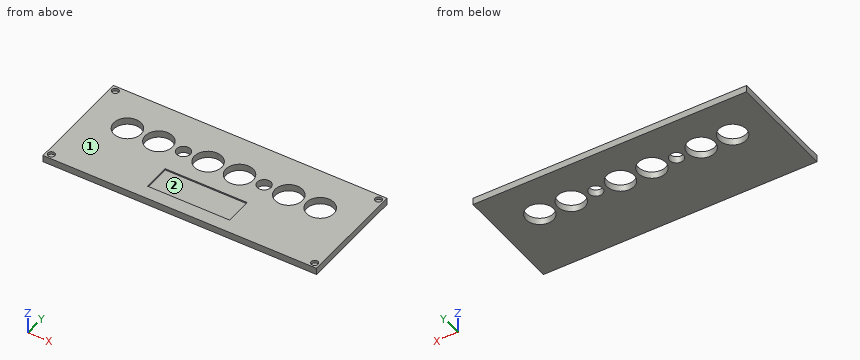
from build123d import *

# Parameters (mm, degrees)
CROQUIS1_W              = 200
CROQUIS1_H              = 80
SALIENTE_EXTRUIR1_DEPTH = 5
CROQUIS2_R              = 2.5
CORTAR_EXTRUIR1_DEPTH   = 2
CROQUIS3_W              = 60
CROQUIS3_H              = 20
CORTAR_EXTRUIR2_DEPTH   = 1
CROQUIS4_R              = 10
CROQUIS4_R_2            = 5
CORTAR_EXTRUIR3_DEPTH   = 5


with BuildPart() as part:
    # Croquis1 → Saliente-Extruir1 (new body)
    with BuildSketch(Plane.XY):
        Rectangle(CROQUIS1_W, CROQUIS1_H)
    extrude(amount=SALIENTE_EXTRUIR1_DEPTH)

    # Croquis2 → Cortar-Extruir1 (cut)
    with BuildSketch(Plane.XY.offset(5)):
        with Locations((-96.25, 36.25)):
            Circle(CROQUIS2_R)
        with Locations((96.25, 36.25)):
            Circle(CROQUIS2_R)
        with Locations((96.25, -36.25)):
            Circle(CROQUIS2_R)
        with Locations((-96.25, -36.25)):
            Circle(CROQUIS2_R)
    extrude(amount=-CORTAR_EXTRUIR1_DEPTH, mode=Mode.SUBTRACT)

    # Croquis3 → Cortar-Extruir2 (cut)
    with BuildSketch(Plane.XY.offset(5)):
        with Locations((0, -20)):
            Rectangle(CROQUIS3_W, CROQUIS3_H)
    extrude(amount=-CORTAR_EXTRUIR2_DEPTH, mode=Mode.SUBTRACT)

    # Croquis4 → Cortar-Extruir3 (cut)
    with BuildSketch(Plane.XY.offset(5)):
        with Locations((-70.5, 10)):
            Circle(CROQUIS4_R)
        with Locations((-47.5, 10)):
            Circle(CROQUIS4_R)
        with Locations((-29.5, 10)):
            Circle(CROQUIS4_R_2)
        with Locations((-11.5, 10)):
            Circle(CROQUIS4_R)
        with Locations((11.5, 10)):
            Circle(CROQUIS4_R)
        with Locations((29.5, 10)):
            Circle(CROQUIS4_R_2)
        with Locations((47.5, 10)):
            Circle(CROQUIS4_R)
        with Locations((70.5, 10)):
            Circle(CROQUIS4_R)
    extrude(amount=-CORTAR_EXTRUIR3_DEPTH, mode=Mode.SUBTRACT)


solid = part.part
Work out the finished part from the listing and answer in its coordinate system (mm). Face numbers are marked on the shaded views. Coordinates: 2 decimals unless noted, no trailing zeros. Loops run counter-clockwise (first coordinate to the right, second up) from the corner with the lowest first, then second, coordinate; pieces in that order, holes last. Notation, with made-up numbers: M 27,-12.5 L 52,-12.5 A29 cw 52,16.5 Z; hole C 14,83.5 d1. An arc over 180 degrees is marked long. Answer in a Markdown table with one row per item. Add a question column.
1. Find section B-B, the plane x = 47.5. Write down the section's boundary in (y, z), then the cut area to 3 significant figures.
2. Find section D-D, the plane x = -96.25. Write down the section's boundary in (y, z), then the cut area to 3 significant figures.
3. The mould has two halves that part along X. Classify the marked faces 1 and 2: pulls with the +X half, pulls with the -X half, needs draft (parallel to the pull), parting line crosses it, or undercut.
4. Find section A-A, the plane z = 0.9. State how many separate pieces and enclosed holes the cut face has, then the cut area to 3 significant figures.
5. Consider L1, parallel to Y at x = 96.25, z = 4.65; L2, parallel to Y at x = -12, z = 4.1; L3, parallel to Y at x = -71, z = 2.45. Determine where each line is inside the solid, lowest interval first.
6. Find section C-C, the plane y = 36.25. Write down the section's boundary in (x, z).
7. Flat-ended cylindrical pins translate along their axes: P1, Ø18, axis at x = 11.5, y = 10, coming from the +Z side; P2, Ø3, axis at x = -26, y = -19.5, coming from the +Z side. Find the tip coordinate at first contact, or state that the pin passes through.
Reported:
| question | item | result |
|---|---|---|
| 1 | outline | M -40,0 L 0,0 L 0,5 L -40,5 Z; M 20,0 L 40,0 L 40,5 L 20,5 Z |
| 1 | area | 300 mm^2 |
| 2 | outline | M -40,0 L 40,0 L 40,5 L 38.75,5 L 38.75,3 L 33.75,3 L 33.75,5 L -33.75,5 L -33.75,3 L -38.75,3 L -38.75,5 L -40,5 Z |
| 2 | area | 380 mm^2 |
| 3 | face 1 | needs draft |
| 3 | face 2 | undercut |
| 4 | separate pieces | 1 |
| 4 | enclosed holes | 8 |
| 4 | area | 14,000 mm^2 |
| 5 | L1 | y = -40 to -38.75, -33.75 to 33.75, 38.75 to 40 |
| 5 | L2 | y = -40 to -30, -10 to 0.01, 19.99 to 40 |
| 5 | L3 | y = -40 to 0.01, 19.99 to 40 |
| 6 | outline | M -100,0 L 100,0 L 100,5 L 98.75,5 L 98.75,3 L 93.75,3 L 93.75,5 L -93.75,5 L -93.75,3 L -98.75,3 L -98.75,5 L -100,5 Z |
| 7 | P1 | passes through |
| 7 | P2 | stops at z = 4 |
